from build123d import *

# Parameters (mm, degrees)
SKETCH_1_W          = 70
SKETCH_1_H          = 30
SKETCH_1_R          = 2.75
EXTRUDE_1_DEPTH     = 5
SKETCH_2_W          = 30
SKETCH_2_H          = 30
EXTRUDE_2_DEPTH     = 20
SKETCH_3_R          = 13
CUT_EXTRUDE_1_DEPTH = 26
EXTRUDE_3_DEPTH     = 4


with BuildPart() as part:
    # 草图1 → 凸台-拉伸1 (new body)
    with BuildSketch(Plane.XY):
        Rectangle(SKETCH_1_W, SKETCH_1_H)
        with Locations((-28, 0)):
            Circle(SKETCH_1_R, mode=Mode.SUBTRACT)
        with Locations((28, 0)):
            Circle(SKETCH_1_R, mode=Mode.SUBTRACT)
    extrude(amount=EXTRUDE_1_DEPTH)

    # 草图2 → 凸台-拉伸2 (add)
    with BuildSketch(Plane.XY.offset(5)):
        Rectangle(SKETCH_2_W, SKETCH_2_H)
    extrude(amount=EXTRUDE_2_DEPTH)

    # 草图3 → 切除-拉伸1 (cut, through all)
    with BuildSketch(Plane.XY.offset(25)):
        Circle(SKETCH_3_R)
    extrude(amount=-CUT_EXTRUDE_1_DEPTH, mode=Mode.SUBTRACT)

    # 草图4 → 凸台-拉伸3 (add)
    with BuildSketch(Plane.XZ.offset(15)):
        Polygon((-15, 25), (-35, 5), (-15, 5), align=None)
        Polygon((15, 25), (15, 5), (35, 5), align=None)
    extrude_3 = extrude(amount=-EXTRUDE_3_DEPTH)

    # 镜向1: 凸台-拉伸3 across plane
    add(extrude_3.mirror(Plane.ZX))


solid = part.part
Source: CAD feature listing. Evaluate the final solid. Frame: model axes, mm. A direction names the side the tool comes from. Give positions to 0.01 mm unless a question says otherwise; leave off trailing zeros. Order: outer loops, then holes, each group sorted by start corner. A loop starts at its lowest first (then second) coordinate and runs counter-clockwise, first axis right, second up. Notation, with made-up numbers: (-8.5, -11) -> (40.5, -11) arc R27 ccw to (40.5, 25) -> close; hole circle Ø3 at (49, 53.5). An arc over 180 degrees is marked (long way). Use a Markdown table: item, result.
1) Contact query for flat-ended pins moving along their axis: P1, Ø6, axis at x = -28.5, y = -3.5, coming from the +Z side; P2, Ø2, axis at x = -22.5, z = 20, coming from the +Y side; P3, Ø10, axis at y = 4.5, z = 15, coming from the +X side; P4, Ø1.5, axis at y = -9, z = 9, coming from the -X side. Output: stop coordinate, or through.
Answer list:
| item | result |
|---|---|
| P1 | z = 5 |
| P2 | through |
| P3 | x = 15 |
| P4 | x = -15 |
2) Mould query, pull axis X, two halves, no side actions, for faces 4 (the flat face through (20, -11, 11)), 5 (the flat face through (35, 0, 2)), 6 (the flat face through (-25, -13, 15)), 7 (the cylindrical face through (25.253, 0.121, 2.465)). Classes: +X half, -X half, draft (parallel to the pull), parting line (faces both ways), or undercut.
Answer list:
| item | result |
|---|---|
| face 4 | draft |
| face 5 | +X half |
| face 6 | -X half |
| face 7 | undercut |
3) Ray query, line 1 along Y through (x, z) = (-28, 3.05); line 2 along Y through (x, z) = (17.5, 14); line 3 along Z through (x, y) = (24.5, 0.5). Return the intervals inside material, ascending. Write a range as [from, to].
Answer list:
| item | result |
|---|---|
| line 1 | [-15, -2.75], [2.75, 15] |
| line 2 | [-15, -11], [11, 15] |
| line 3 | [0, 5] |
4) Section query A-A, the plane x = 0. Return the cut outline in (y, z).
Answer list:
| item | result |
|---|---|
| outline | (-15, 0) -> (-13, 0) -> (-13, 25) -> (-15, 25) -> close; (13, 0) -> (15, 0) -> (15, 25) -> (13, 25) -> close |
5) Section query B-B, the plane y = 0. Return the cut outline in (x, z), then the cut area to 3 significant figures.
Answer list:
| item | result |
|---|---|
| outline | (-35, 0) -> (-30.75, 0) -> (-30.75, 5) -> (-35, 5) -> close; (-25.25, 0) -> (-13, 0) -> (-13, 25) -> (-15, 25) -> (-15, 5) -> (-25.25, 5) -> close; (13, 0) -> (25.25, 0) -> (25.25, 5) -> (15, 5) -> (15, 25) -> (13, 25) -> close; (30.75, 0) -> (35, 0) -> (35, 5) -> (30.75, 5) -> close |
| area | 245 mm² |
6) Section query D-D, the plane y = 9.5. Return the cut outline in (x, z), then the cut area to 3 significant figures.
Answer list:
| item | result |
|---|---|
| outline | (-35, 0) -> (-8.87, 0) -> (-8.87, 25) -> (-15, 25) -> (-15, 5) -> (-35, 5) -> close; (8.87, 0) -> (35, 0) -> (35, 5) -> (15, 5) -> (15, 25) -> (8.87, 25) -> close |
| area | 506 mm² |
7) Reachability of faces 1 (the flat face through (15, 0, 15)), 2 (the cylindrical face through (-10.316, -7.91, 12.675)), 3 (the flat face through (-15, 0, 15)) from +Z, -Z, +X, -X, +Y, -Y: full face, straight path, thin tool, end or side. Return the list, or none.
Answer list:
| item | result |
|---|---|
| face 1 | +Z, +X |
| face 2 | +Z, -Z |
| face 3 | +Z, -X |
8) Section query C-C, the plane z = 6. Return the cut outline in (x, y), then the cut area to 3 significant figures.
Answer list:
| item | result |
|---|---|
| outline | (-34, -15) -> (34, -15) -> (34, -11) -> (15, -11) -> (15, 11) -> (34, 11) -> (34, 15) -> (-34, 15) -> (-34, 11) -> (-15, 11) -> (-15, -11) -> (-34, -11) -> close; hole circle Ø26 at (0, 0) |
| area | 673 mm² |
